from build123d import *

# Parameters (mm, degrees)
F1_DEPTH  = 3.175
F2_SIZE   = 101.6
F4_D      = 14.2875
F5_W      = 85.852
F5_H      = 25.4
F5_W_2    = 507.99026
F6_DEPTH  = 6.35
F8_D      = 20.6375
F11_DEPTH = 6.35
F12_R     = 25.4


with BuildPart() as f1:
    # F0 (on Front) → F1 (new body, symmetric)
    with BuildSketch(Plane.XZ):
        with BuildLine():
            Line((-692.15, 171.45), (-692.15, 0))
            Line((-692.15, 0), (-107.95, 0))
            Line((-107.95, 0), (-107.95, 45.974))
            ThreePointArc((-107.95, 45.974), (-104.230256, 54.954256), (-95.25, 58.674))
            Line((-95.25, 58.674), (95.25, 58.674))
            ThreePointArc((95.25, 58.674), (104.230256, 54.954256), (107.95, 45.974))
            Line((107.95, 45.974), (107.95, 0))
            Line((107.95, 0), (193.802, 0))
            Line((193.802, 0), (193.802, 120.65))
            ThreePointArc((193.802, 120.65), (178.923024, 156.571024), (143.002, 171.45))
            Line((143.002, 171.45), (-692.15, 171.45))
        make_face()
    extrude(amount=F1_DEPTH, both=True)

    # F2
    f2_edges = [f1.edges().sort_by_distance(p)[0] for p in [
        (-692.15, 0, 171.45),
    ]]
    chamfer(f2_edges, length=F2_SIZE)

    # F4 (through all)
    with Locations(Plane.XZ.offset(3.175)):
        with Locations((-610.616, 41.402), (-663.448, 51.562)):
            Hole(F4_D / 2)

    # F5 (on Top) → F6 (join)
    with BuildSketch(Plane.XY):
        with Locations((150.876, -3.175)):
            Rectangle(F5_W, F5_H)
        with Locations((-361.94513, -3.175)):
            Rectangle(F5_W_2, F5_H)
        with BuildLine():
            Line((-107.95, -15.875), (-615.94026, -15.875))
            Line((-615.94026, -15.875), (-190.49026, -114.427))
            Line((-190.49026, -114.427), (-143.002, -114.427))
            ThreePointArc((-143.002, -114.427), (-118.216493, -104.160507), (-107.95, -79.375))
            Line((-107.95, -79.375), (-107.95, -15.875))
        make_face()
        with BuildLine():
            Line((193.802, -15.875), (107.95, -15.875))
            Line((107.95, -15.875), (107.95, -79.375))
            ThreePointArc((107.95, -79.375), (118.216493, -104.160507), (143.002, -114.427))
            Line((143.002, -114.427), (193.802, -114.427))
            Line((193.802, -114.427), (193.802, -15.875))
        make_face()
    extrude(amount=-F6_DEPTH)

    # F8 (through all)
    with Locations(Plane.XY):
        with Locations((-139.7, -79.375), (139.7, -79.375)):
            Hole(F8_D / 2)

    # F10 (on offset) → F11 (join)
    with BuildSketch(Plane.YZ.offset(-403.352)):
        Polygon((-53.975, 0), (-3.175, 0), (-3.175, 152.4), (-15.875, 152.4), (-53.975, 19.05), align=None)
    extrude(amount=-F11_DEPTH)

    # F12
    f12_edges = [f1.edges().sort_by_distance(p)[0] for p in [
        (-692.15, 0, 0),
    ]]
    fillet(f12_edges, radius=F12_R)


solid = f1.part
Input: part model. Units: mm. Frame: model coordinates. A direction names the side the tool comes from. Round coordinates to 2 decimals unless told otherwise and drop trailing zeros. Write each loop counter-clockwise with the first axis right and the second up, starting at its lowest first coordinate (ties: lowest second). Pieces come first, ordered by that corner, then holes.
1) Cut plane C-C (z = 144). Return the cut outline in (x, y) (3 decimals).
2) Cut plane B-B (x = -361). Return the cut outline in (y, z) (3 decimals), then the cut area to 4 significant figures.
3) Cut plane D-D (y = -41.5). Return the cut outline in (x, z), then the cut area to 3 significant figures.
4) Cut plane A-A (y = -99.5). Return the cut outline in (x, z).
5) Contact query for flat-ended pins moving along their axis: P1, Ø5, axis at x = -553.5, z = 67, coming from the +Y side (3 decimals); P2, Ø1.5, axis at y = -6, z = 75.5, coming from the -X side; P3, Ø1.9, axis at x = -407, z = 6.5, coming from the -Y side (3 decimals). Output: stop coordinate, or through.
6) Reachability of faces 5 (the flat face through (-255, 3.175, 87)), 6 (the flat face through (107.95, -22, -1)), 7 (the cylindrical face through (117.95, -103.89, -3.13)), 8 (the flat face through (150, -58, 0)) from +Z, -Z, +X, -X, +Y, -Y: full face, straight path, thin tool, end or side. Return the list, or none.
7) Ray query, L1, parallel to Y at x = -139.7, z = -2 (3 decimals); L2, parallel to Z at x = -382.5, y = -13.5; L3, parallel to Y at x = -144.5, z = 10.5 (3 decimals). Return the intervals inside material, ascending.
8) Draft query along Z for faces 1 (the cylindrical face through (179.32, -0.04, 156.17)), 2 (the flat face through (-255, -3.175, 87)), 3 (the cylindrical face through (-656.31, 0.04, 51.88)), 4 (the cylindrical face through (-604.947, 0.044, 37.055)). Return one class per face: pulls with the +Z half, pulls with the -Z half, needs draft (parallel to the pull), parting line crosses it, or undercut.
Geometry says:
1. outline: (-618, -3.175) - (-409.702, -3.175) - (-409.702, -18.275) - (-403.352, -18.275) - (-403.352, -3.175) - (188.118, -3.175) - (188.118, 3.175) - (-618, 3.175) - close
2. outline: (-74.93, -6.35) - (9.525, -6.35) - (9.525, 0) - (3.175, 0) - (3.175, 171.45) - (-3.175, 171.45) - (-3.175, 0) - (-74.93, 0) - close
2. area: 1,625 mm2
3. outline: (-505.32, -6.35) - (-107.95, -6.35) - (-107.95, 0) - (-403.35, 0) - (-403.35, 62.71) - (-409.7, 62.71) - (-409.7, 0) - (-505.32, 0) - close; (107.95, -6.35) - (193.8, -6.35) - (193.8, 0) - (107.95, 0) - close
3. area: 3,470 mm2
4. outline: (-254.93, -6.35) - (-114.3, -6.35) - (-114.3, 0) - (-254.93, 0) - close; (114.3, -6.35) - (193.8, -6.35) - (193.8, 0) - (114.3, 0) - close
5. P1: stops at y = 3.175
5. P2: stops at x = -409.7
5. P3: stops at y = -53.975
6. face 5: +Z, +X, -X, +Y
6. face 6: -Z, +Y, -Y
6. face 7: +Z, -Z, -Y
6. face 8: +Z, +X, -Y
7. L1: y = -114.271 to -89.694, -69.056 to 9.525
7. L2: z = -6.35 to 0
7. L3: y = -3.175 to 3.175
8. face 1: pulls with the +Z half
8. face 2: needs draft
8. face 3: undercut
8. face 4: undercut
